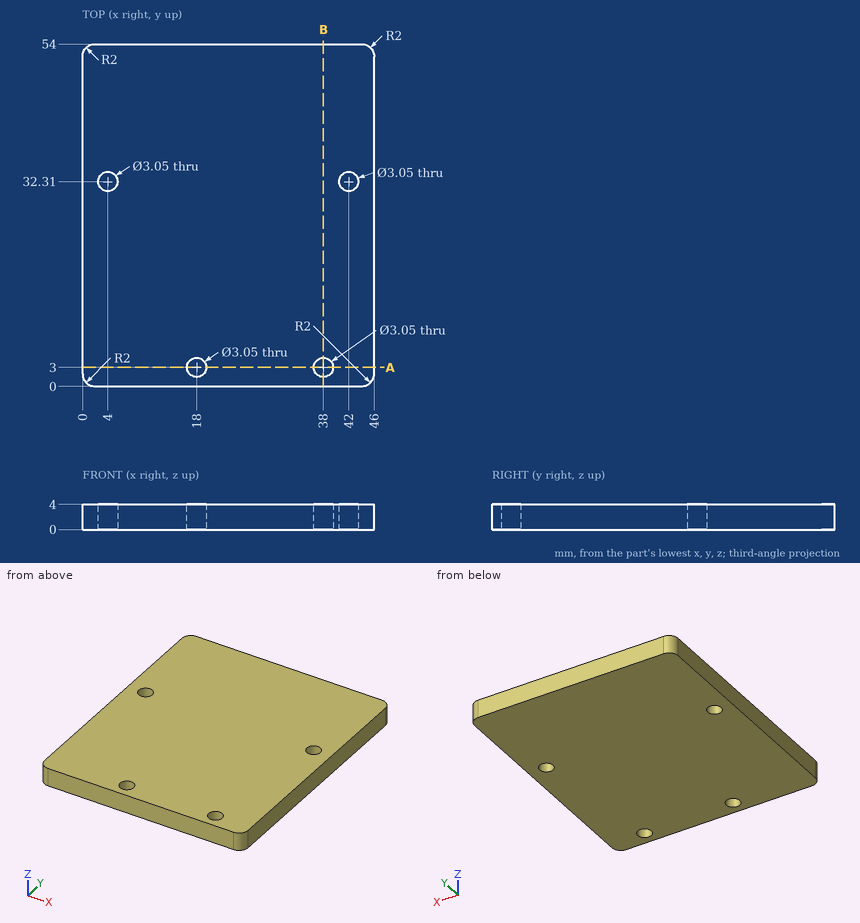
The figure shows three views and two pictorial views of one solid part (mm, origin at its lowest corner). Answer the questions. Round coordinates to 2 decimals unless told otherwise and drop trailing zeros. Write each loop counter-clockwise with the first axis right and the second up, starting at its lowest first coordinate (ties: lowest second). Pieces come first, ordered by that corner, then holes. Notation, with made-up numbers: (18, 89) - (50, 89) arc R25 cw to (50, 128) - close; hole circle Ø1 at (42, 7). An arc over 180 degrees is marked (long way). Answer in a Markdown table with one row per item. Add a question column.
1. Given pin 1 (4 mm diameter, centred on x = 18, y = 3, fed in from -Z); pin 2 (1.8 mm diameter, centred on x = 38, y = 3, fed in from -Z), each flat-ended and moving along its own axis, determine where each tip first touches the part or whether it passes through.
2. Find the intervals of material crossed by line 1 along Y through (x, z) = (38, 0.9) (1 decimal); line 2 along Y through (x, z) = (4, 1.35) (1 decimal), in increasing order. Write a range as from..to.
3. A cutting plane is placed at A-A, the plane y = 3. Determine the outline of the cut face in (x, z) (1 decimal), and give its area (3 significant figures).
4. A cutting plane is placed at B-B, the plane x = 38. Determine the outline of the cut face in (y, z) (1 decimal).
Worked out:
| question | item | result |
|---|---|---|
| 1 | pin 1 | z = 0 |
| 1 | pin 2 | through |
| 2 | line 1 | 0..1.5, 4.5..54 |
| 2 | line 2 | 0..30.8, 33.8..54 |
| 3 | outline | (0, 0) - (16.5, 0) - (16.5, 4) - (0, 4) - close; (19.5, 0) - (36.5, 0) - (36.5, 4) - (19.5, 4) - close; (39.5, 0) - (46, 0) - (46, 4) - (39.5, 4) - close |
| 3 | area | 160 mm^2 |
| 4 | outline | (0, 0) - (1.5, 0) - (1.5, 4) - (0, 4) - close; (4.5, 0) - (54, 0) - (54, 4) - (4.5, 4) - close |
